Verification items for the finished model (mm, model axes). A direction names the side the tool comes from. Round coordinates to 2 decimals unless told otherwise and drop trailing zeros. Order: outer loops, then holes, each group sorted by start corner. A loop starts at its lowest first (then second) coordinate and runs counter-clockwise, first axis right, second up. Notation, with made-up numbers: M 24.25,-26 L 76.25,-26 A31 ccw 76.25,7 Z; hole C 29.5,34.25 d8. An arc over 180 degrees is marked long. One line per item, written item: value. Start each with the question number.
from build123d import *

# Parameters (mm, degrees)
SKETCH1_R           = 6.85
BOSS_EXTRUDE1_DEPTH = 11.8
BOSS_EXTRUDE2_DEPTH = 5
SKETCH3_R           = 5
BOSS_EXTRUDE3_DEPTH = 3
SKETCH4_R           = 12
BOSS_EXTRUDE4_DEPTH = 47.2
SKETCH5_R           = 6
BOSS_EXTRUDE5_DEPTH = 9


with BuildPart() as part:
    # Sketch1 → Boss-Extrude1 (new body)
    with BuildSketch(Plane(origin=(0, 0, 0), x_dir=(1, 0, 0), z_dir=(0, 1, 0))):
        Circle(SKETCH1_R)
    extrude(amount=BOSS_EXTRUDE1_DEPTH)

    # Sketch2 → Boss-Extrude2 (add)
    with BuildSketch(Plane(origin=(0, 11.8, 0), x_dir=(1, 0, 0), z_dir=(0, 1, 0))):
        Polygon((0, 10.392304845), (-9, 5.196152423), (-9, -5.196152423), (0, -10.392304845), (9, -5.196152423), (9, 5.196152423), align=None)
    extrude(amount=BOSS_EXTRUDE2_DEPTH)

    # Sketch3 → Boss-Extrude3 (add)
    with BuildSketch(Plane(origin=(0, 16.8, 0), x_dir=(1, 0, 0), z_dir=(0, 1, 0))):
        Circle(SKETCH3_R)
    extrude(amount=BOSS_EXTRUDE3_DEPTH)

    # Sketch4 → Boss-Extrude4 (add)
    with BuildSketch(Plane(origin=(0, 19.8, 0), x_dir=(1, 0, 0), z_dir=(0, 1, 0))):
        Circle(SKETCH4_R)
    extrude(amount=BOSS_EXTRUDE4_DEPTH)

    # Sketch5 → Boss-Extrude5 (add)
    with BuildSketch(Plane(origin=(0, 67, 0), x_dir=(1, 0, 0), z_dir=(0, 1, 0))):
        Circle(SKETCH5_R)
    extrude(amount=BOSS_EXTRUDE5_DEPTH)


solid = part.part
1. Tool access check on faces 1 (the face through (-4.44, 14.26, -7.83)), 2 (the face through (-9, 14, 0)), 3 (the face through (-1.08, 18.28, 4.88)). Record the directions out of +Z, -Z, +X, -X, +Y, -Y that give a thin tool (end or side, any length) a straight path to the whole face; none if there is none.
2. Section check B-B (x = -8). Record the cut outline in (y, z).
3. Section check C-C (z = 8.75). Record the cut outline in (x, y), and give its area (3 significant figures).
4. Depth check by flat-ended pin: pin 1 (5 mm diameter, centred on y = 22.5, z = -7.5, fed in from +X); pin 2 (1.5 mm diameter, centred on y = 14, z = 2, fed in from -X); pin 3 (2 mm diameter, centred on x = 7, z = 8.5, fed in from +Y). Enter the tip coordinate at first touch or a pass-through.
5. Scan lines: line 1 along Y through (x, z) = (5.75, -4); line 2 along Y through (x, z) = (-8.75, -7.25); line 3 along Y through (x, z) = (0.75, -5.25). Record each from-to range of solid material in increasing order.
6. Draft check along Y on faces 4 (the face through (0, 11.8, 7)), 5 (the face through (-2, 16.8, -5)), 6 (the face through (0, 76, 0)). Enter one of: released by +Y, released by -Y, zero draft, split by the parting line, or undercut.
7. Section check D-D (y = 8.5). Record the cut outline in (x, z).
8. Section check A-A (z = 0). Record the cut outline in (x, y), and give its area (3 significant figures).
Geometry check:
1. face 1: -Z, -X, -Y
1. face 2: +Z, -Z, -X, -Y
1. face 3: none
2. outline: M 11.8,-5.77 L 16.8,-5.77 L 16.8,5.77 L 11.8,5.77 Z; M 19.8,-8.94 L 67,-8.94 L 67,8.94 L 19.8,8.94 Z
3. outline: M -8.21,19.8 L 8.21,19.8 L 8.21,67 L -8.21,67 Z; M -2.84,11.8 L 2.84,11.8 L 2.84,16.8 L -2.84,16.8 Z
3. area: 804 mm²
4. pin 1: stops at x = 10.91
4. pin 2: stops at x = -9
4. pin 3: stops at y = 67
5. line 1: y = 11.8 to 16.8, 19.8 to 67
5. line 2: y = 19.8 to 67
5. line 3: y = 0 to 16.8, 19.8 to 76
6. face 4: released by -Y
6. face 5: undercut
6. face 6: released by +Y
7. outline: C 0,0 d13.7
8. outline: M -12,19.8 L -5,19.8 L -5,16.8 L -9,16.8 L -9,11.8 L -6.85,11.8 L -6.85,0 L 6.85,0 L 6.85,11.8 L 9,11.8 L 9,16.8 L 5,16.8 L 5,19.8 L 12,19.8 L 12,67 L 6,67 L 6,76 L -6,76 L -6,67 L -12,67 Z
8. area: 1,520 mm²
